Solid Edge part; units mm, degrees
sketch "Sketch1" plane through (0, 0, 0) normal (1, 0, 0) x (0, 1, 0)
  line L0 (-5, 20) -> (-2, 20)
  line L1 (-2, 20) -> (-2, -20)
  line L2 (-2, -20) -> (-5, -20)
  line L3 (-5, -20) -> (-5, 20)
  line L4 (-7.5, 23) -> (0, 23)
  line L5 (0, 23) -> (0, -23)
  line L6 (0, -23) -> (-7.5, -23)
  line L7 (-7.5, -23) -> (-7.5, 23)
extrude "Protrusion1" add sketch "Sketch1" against normal blind 6
sketch "Sketch2" plane through (0, 0, 0) normal (0, -1, 0) x (1, 0, 0)
  line L0 (-12.4, 15.6) -> (3, 15.6)
  line L1 (3, 15.6) -> (3, 23)
  line L2 (3, 23) -> (-12.4, 23)
  line L3 (-12.4, 23) -> (-12.4, 15.6)
  circle A0 centre (-9.2, 19.3) radius 1.7
  line L4 (3, -23) -> (-12.4, -23)
  line L5 (-12.4, -23) -> (-12.4, -15.6)
  line L6 (-12.4, -15.6) -> (3, -15.6)
  line L7 (3, -15.6) -> (3, -23)
  circle A1 centre (-9, -19.5) radius 1.5
extrude "Protrusion2" add sketch "Sketch2" along normal up to surface (2 mm away)
fillet "Round_1" radius 1 6 edges at (-6, -5, 0) (-6, -7.5, 0) (0, -7.5, 0) (0, -2, 0) (0, -2, 21.5) (0, -2, -21.5)
fillet "Round_2" radius 2 6 edges at (-12.4, -1, 23) (-12.4, -1, 15.6) (-12.4, -1, -15.6) (-12.4, -1, -23) (3, -2, 19.3) (3, -2, -19.3)
sketch "Sketch3" plane through (0, 0, 0) normal (0, -1, 0) x (1, 0, 0)
  line L0 (-20.672, -15.6) -> (-20.672, 15.6)
  line L1 (-20.672, 15.6) -> (17.3564, 15.6)
  line L2 (17.3564, 15.6) -> (17.3564, -15.6)
  line L3 (17.3564, -15.6) -> (-20.672, -15.6)
extrude "Cutout1" cut sketch "Sketch3" along normal up to next
The listing builds one solid part. Answer for the finished solid, in the listing's coordinates (mm). A direction names the side the tool comes from. Coordinates: 2 decimals unless noted, no trailing zeros. Write each loop counter-clockwise with the first axis right and the second up, starting at its lowest first coordinate (ties: lowest second). Pieces come first, ordered by that corner, then holes. Notation, with made-up numbers: M -33,50 L 22,50 A21 cw 22,66 Z; hole C -21,-9 d5. An arc over 180 degrees is marked long. Put each result on its own line as item: value. Start each with the question number.
1. Which of the six approach directions +Z, -Z, +X, -X, +Y, -Y give full straight-line access (tool end or side, diameter ignored) to faces 4 (the flat face through (-6, -6.3, 0.1)), 5 (the flat face through (-2, -5, 0)), 6 (the flat face through (-6, -2, -19)), 7 (the cylindrical face through (-11.83, -1.01, 16.2)), 8 (the cylindrical face through (2.43, -1.4, -19.35))?
2. For a pull along Z with two mould halves and no side action, classify faces 1 (the flat face through (-12.4, -1, -19)), 2 (the flat face through (-4, -1, -15.6)), 3 (the cylindrical face through (-11.83, -1.01, -22.4)) as pulls with the +Z half, pulls with the -Z half, needs draft (parallel to the pull), parting line crosses it, or undercut.
3. A cutting plane is placed at D-D on y = -1.5. Write down the section's boundary in (x, z), then the cut area to 3 significant figures.
4. Flat-ended cylindrical pins translate along their axes: P1, Ø3, axis at y = -5, z = 5, coming from the +X side; P2, Ø2, axis at y = -5, z = 1.5, coming from the -X side; P3, Ø4, axis at x = -3.5, z = -8.5, coming from the +Y side. Find the tip coordinate at first contact, or state that the pin passes through.
5. A cutting plane is placed at B-B on y = -4. Write down the section's boundary in (x, z).
6. A cutting plane is placed at C-C on x = -6.5. Write down the section's boundary in (y, z).
7. Consider line 1 (Z direction, x = -1.25, y = -2.5); line 2 (Z direction, x = -9, y = -1); line 3 (Z direction, x = -1, y = -0.5). Determine where each line is inside the solid, lowest interval first. Write a range as from..to.
8. A cutting plane is placed at A-A on z = 19.3. Count the separate pieces of the cut face and the enclosed holes in it, then the cut area to 3 significant figures.
Resolved:
1. face 4: +Z, -Z, -X, -Y
1. face 5: +X, -X
1. face 6: -X
1. face 7: -X, +Y, -Y
1. face 8: +Z, -Z, +X, -Y
2. face 1: needs draft
2. face 2: undercut
2. face 3: pulls with the -Z half
3. outline: M -12.4,-21 A2 ccw -10.4,-23 L 2.32,-23 L 2.32,-15.6 L -10.4,-15.6 A2 ccw -12.4,-17.6 Z; M -12.4,17.6 A2 ccw -10.4,15.6 L 2.32,15.6 L 2.32,23 L -10.4,23 A2 ccw -12.4,21 Z; hole C -9.2,19.3 d3.4; hole C -9,-19.5 d3
3. area: 198 mm2
4. P1: stops at x = 0
4. P2: stops at x = -6
4. P3: stops at y = -5
5. outline: M -6,-23 L 0,-23 L 0,-20 L -6,-20 Z; M -6,20 L 0,20 L 0,23 L -6,23 Z
6. outline: M -2,-23 L 0,-23 L 0,-15.6 L -2,-15.6 Z; M -2,15.6 L 0,15.6 L 0,23 L -2,23 Z
7. line 1: z = -23..-20, 20..23
7. line 2: z = -23..-21, -18..-15.6, 15.6..17.61, 20.99..23
7. line 3: z = -23..-15.6, 15.6..23
8. separate pieces: 3
8. enclosed holes: 0
8. area: 37.5 mm2
